```python
from build123d import *

# Parameters (mm, degrees)
F1_DEPTH = 1981.2
F3_DEPTH = 152.4
F5_DEPTH = 152.4


with BuildPart() as f1:
    # F0 (on Front) → F1 (new body)
    with BuildSketch(Plane.XZ):
        with BuildLine():
            Line((0, 152.4), (0, 0))
            Line((0, 0), (20.955, 0))
            Line((20.955, 0), (20.955, 136.525))
            ThreePointArc((20.955, 136.525), (17.14516, 145.595503), (8.001, 149.225))
            Line((8.001, 149.225), (8.001, 152.4))
            Line((8.001, 152.4), (0, 152.4))
        make_face()
    extrude(amount=-F1_DEPTH)

    # F2 (on face) → F3 (cut)
    with BuildSketch(Plane(origin=(0, 0, 0), x_dir=(1, 0, 0), z_dir=(0, 0, -1))):
        Polygon((0, -20.955), (20.955, 0), (0, 0), align=None)
    extrude(amount=-F3_DEPTH, mode=Mode.SUBTRACT)

    # F4 (on face) → F5 (cut)
    with BuildSketch(Plane(origin=(0, 0, 0), x_dir=(1, 0, 0), z_dir=(0, 0, -1))):
        Polygon((0, -1981.2), (20.955, -1981.2), (0, -1960.245), align=None)
    extrude(amount=-F5_DEPTH, mode=Mode.SUBTRACT)


solid = f1.part
```
Work out the finished part from the listing and answer in its coordinate system (mm). Give positions to 0.01 mm unless a question says otherwise; leave off trailing zeros. Loops run counter-clockwise (first coordinate to the right, second up) from the corner with the lowest first, then second, coordinate; pieces in that order, holes last. Notation, with made-up numbers: (-1, 53.5) -> (12, 53.5) arc R11 cw to (12, 71.5) -> close; hole circle Ø9 at (72.25, 38.5). An arc over 180 degrees is marked (long way). One line per question, with ' | ' between items. Start each with the question number.
1) Section A-A, the plane y = 1007 is taken. Determine the outline of the cut face in (x, z) (1 decimal), then the cut area to 3 significant figures.
2) Straight lines are drawn through the part: L1, parallel to Z at x = 9.25, y = 958; L2, parallel to Z at x = 9.75, y = 1258.5; L3, parallel to Y at x = 1.5, z = 78.5 (3 decimals). For each, find the intervals that lie inside material, in ascending order.
3) Each of these flat-tipped pins is pushed along its axis until it touches: pin 1 (3 mm diameter, centred on y = 266, z = 104.5, fed in from -X); pin 2 (3 mm diameter, centred on x = 9.5, z = 40.5, fed in from +Y) (3 decimals); pin 3 (1.6 mm diameter, centred on y = 684, z = 151.5, fed in from +X); pin 4 (4 mm diameter, centred on x = 9.5, z = 82.5, fed in from +Y) (3 decimals). Where does it stop, or does it pass through?
4) Section B-B, the plane x = 15.5 is taken. Determine the outline of the cut face in (y, z) (3 decimals).
Resolved:
1) outline: (0, 0) -> (21, 0) -> (21, 136.5) arc R12.7 ccw to (8, 149.2) -> (8, 152.4) -> (0, 152.4) -> close | area: 3,120 mm2
2) L1: 0 to 149.19 | L2: 0 to 149.14 | L3: 19.455 to 1961.745
3) pin 1: x = 0 | pin 2: y = 1971.245 | pin 3: x = 8 | pin 4: y = 1971.745
4) outline: (5.455, 0) -> (1975.745, 0) -> (1975.745, 146.957) -> (5.455, 146.957) -> close
